Design review of the part built by this model. Coordinates are the model's own, in mm. Face numbers are marked on the shaded views. A direction names the side the tool comes from. Give positions to 0.01 mm unless a question says otherwise; leave off trailing zeros. Order: outer loops, then holes, each group sorted by start corner. A loop starts at its lowest first (then second) coordinate and runs counter-clockwise, first axis right, second up. Notation, with made-up numbers: (6.5, 72) -> (13.5, 72) arc R22 cw to (13.5, 78) -> close; hole circle Ø2 at (79.5, 17.25). An arc over 180 degrees is marked (long way). One line per item, written item: value. Start each with the question number.
1) Wall thickness on line 1 along Y through (x, z) = (80, 52); line 2 along Y through (x, z) = (7, 39); line 3 along X through (y, z) = (13, 19) (3 decimals): over which ranges is each line inside the solid? List them lowest first. Write a range as from..to.
2) The part is to be moulded in two halves that separate along X. For the marked faces 6, 7 and 8, say which applies: released by +X, released by -X, zero draft, split by the parting line, or undercut.
3) Consider section A-A (x = 80). State the section outline as (y, z) points (3 decimals), plus the area to 3 significant figures.
4) For pin 1 (15 mm diameter, centred on x = 78.5, y = -5.5, fed in from -Z); pin 2 (15.5 mm diameter, centred on x = 45.5, z = 33, fed in from +Y); pin 3 (5 mm diameter, centred on y = -19, z = 45.5, fed in from -X), all flat-tipped, find the tip position at first contact; note any pin that passes through.
5) Tool access review of the marked faces 1, 2, 3, 4 and 5: name each direction out of +Z, -Z, +X, -X, +Y, -Y from which nothing blocks a thin tool from reaching the whole face with its end or side.
from build123d import *

# Parameters (mm, degrees)
F1_DEPTH = 63.5
F1_TAPER = -3
F0_W     = 25.4
F0_H     = 19.05
F2_DEPTH = 25.4
F3_DEPTH = 7.9375
F5_R     = 5.08


with BuildPart() as f1:
    # F0 (on Front) → F1 (new body, symmetric)
    with BuildSketch(Plane.XZ):
        Polygon((22.225, 9.525), (-41.275, 9.525), (-41.275, -9.525), (41.275, -9.525), (41.275, 9.525), align=None)
    extrude(amount=F1_DEPTH, both=True, taper=F1_TAPER)

    # F0 (on Front) → F2 (join, symmetric)
    with BuildSketch(Plane.XZ):
        with BuildLine():
            Line((22.225, 27.0002), (22.225, 9.525))
            Line((22.225, 9.525), (41.275, 9.525))
            Line((41.275, 9.525), (41.275, 27.0002))
            ThreePointArc((41.275, 27.0002), (45.9246798487, 38.2255201513), (57.15, 42.8752))
            Line((57.15, 42.8752), (60.325, 42.8752))
            Line((60.325, 42.8752), (60.325, 61.9252))
            Line((60.325, 61.9252), (57.15, 61.9252))
            add(Edge.make_bspline(
                [(53.8854342407, 61.7722898912), (54.9842067368, 61.8365871986), (56.0728453275, 61.8876096574), (57.15, 61.9252)],
                knots=[108.5245810491, 108.5245810491, 108.5245810491, 108.5245810491, 111.5045361635, 111.5045361635, 111.5045361635, 111.5045361635], degree=3))
            ThreePointArc((53.8854342407, 61.7722898912), (31.3258777096, 50.5133948686), (22.225, 27.0002))
        make_face()
        with Locations((73.025, 52.4002)):
            Rectangle(F0_W, F0_H)
    extrude(amount=F2_DEPTH, both=True)

    # F0 (on Front) → F3 (join, symmetric)
    with BuildSketch(Plane.XZ):
        with BuildLine():
            add(Edge.make_bspline(
                [(-41.275, 9.525), (-39.5856284224, 39.4828766469), (13.870125209, 59.4306981306), (53.8854342407, 61.7722898912)],
                knots=[0, 0, 0, 0, 108.5245810491, 108.5245810491, 108.5245810491, 108.5245810491], degree=3))
            Line((-41.275, 9.525), (22.225, 9.525))
            Line((22.225, 9.525), (22.225, 27.0002))
            ThreePointArc((22.225, 27.0002), (31.3258777096, 50.5133948686), (53.8854342407, 61.7722898912))
        make_face()
    extrude(amount=F3_DEPTH, both=True)

    # F0 (on Front) → F4 (revolve)
    with BuildSketch(Plane.XZ):
        Polygon((85.725, 66.675), (85.725, 61.9252), (85.725, 42.8752), (85.725, 38.1), (111.125, 38.1), (111.125, 66.675), align=None)
    revolve(axis=Axis((85.725, 0, 52.3875), (0, 0, 1)))

    # F5
    f5_edges = [f1.edges().sort_by_distance(p)[0] for p in [
        (44.602894, -63.5, 0),
        (-44.602894, -63.5, 0),
        (44.602894, 63.5, 0),
        (-44.602894, 63.5, 0),
    ]]
    fillet(f5_edges, radius=F5_R)


solid = f1.part
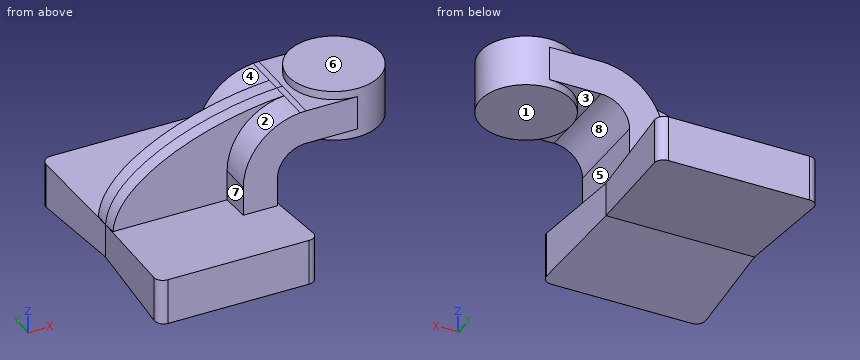
Checked values:
1. line 1: y = -25.4..25.4
1. line 2: y = -7.94..7.94
1. line 3: x = 22.225..41.275
2. face 6: zero draft
2. face 7: released by -X
2. face 8: undercut
3. outline: (-25.4, 42.875) -> (-24.746, 42.875) -> (-24.746, 38.1) -> (24.746, 38.1) -> (24.746, 42.875) -> (25.4, 42.875) -> (25.4, 61.925) -> (24.746, 61.925) -> (24.746, 66.675) -> (-24.746, 66.675) -> (-24.746, 61.925) -> (-25.4, 61.925) -> close
3. area: 1,440 mm^2
4. pin 1: stops at z = 38.1
4. pin 2: stops at y = 25.4
4. pin 3: stops at x = 26.11
5. face 1: -Z, +X, +Y, -Y
5. face 2: +Z, -X, -Y
5. face 3: -Z
5. face 4: +Z, -X, +Y
5. face 5: +X
